Geometry check sheet. Reference: the model listing, model coordinates, mm. Face numbers are marked on the shaded views. A direction names the side the tool comes from. Coordinates: 2 decimals unless noted, no trailing zeros. Loops run counter-clockwise (first coordinate to the right, second up) from the corner with the lowest first, then second, coordinate; pieces in that order, holes last. Notation, with made-up numbers: M 5,66.25 L 38,66.25 A16 cw 38,87.25 Z; hole C 34.25,81.25 d5. An arc over 180 degrees is marked long. Use CSV: the item, a comma, the result in double quotes.
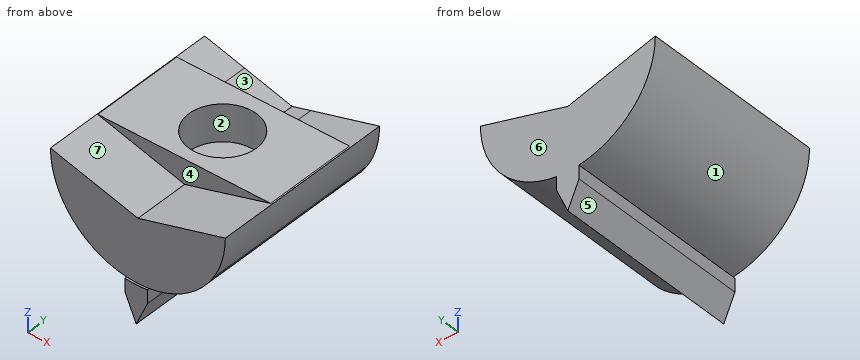
```python
from build123d import *

# Parameters (mm, degrees)
F1_DEPTH = 127
F3_DEPTH = 128.4378021955
F5_DEPTH = 88.5605067015
F6_DEPTH = 23.5462002456
F7_R     = 23.3912457605
F8_DEPTH = 25.4


with BuildPart() as f1:
    # F0 (on Front) → F1 (new body)
    with BuildSketch(Plane.XZ):
        with BuildLine():
            Line((0.0581891033, -16.9071952176), (-60.6434829533, 0))
            ThreePointArc((-60.6434829533, 0), (-58.419745585, -16.2716117976), (-51.9116180406, -31.3498953286))
            Line((-51.9116180406, -31.3498953286), (0.0581891033, -16.9071952176))
        make_face()
        with BuildLine():
            Line((51.9116180406, -31.3498953286), (-51.9116180406, -31.3498953286))
            ThreePointArc((-51.9116180406, -31.3498953286), (0, -60.6434829533), (51.9116180406, -31.3498953286))
        make_face()
        Polygon((0.0581891033, -16.9071952176), (-51.9116180406, -31.3498953286), (51.9116180406, -31.3498953286), align=None)
        with BuildLine():
            Line((60.6434423053, -0.0702144545), (0.0581891033, -16.9071952176))
            Line((0.0581891033, -16.9071952176), (51.9116180406, -31.3498953286))
            ThreePointArc((51.9116180406, -31.3498953286), (58.4103159662, -16.3054289561), (60.6434423053, -0.0702144545))
        make_face()
    extrude(amount=F1_DEPTH)

    # F2 (on face) → F3 (join)
    with BuildSketch(Plane(origin=(0, 0, 0), x_dir=(-1, 0, 0), z_dir=(0, 1, 0))):
        with BuildLine():
            Line((-7.8074381221, -60.1388055641), (-7.8074381221, -69.4347918034))
            Line((-7.8074381221, -69.4347918034), (7.6910599156, -69.4347918034))
            Line((7.6910599156, -69.4347918034), (7.6910599156, -60.1537997311))
            ThreePointArc((7.6910599156, -60.153799731), (-0.0586700775, -60.6434545729), (-7.8074381221, -60.1388055641))
        make_face()
        Polygon((7.6910599156, -69.4347918034), (-7.8074381221, -69.4347918034), (-0.0581891033, -86.9502127171), align=None)
    extrude(amount=-F3_DEPTH)

    # F4 (on Front) → F5 (join)
    with BuildSketch(Plane.XZ):
        Polygon((59.6265792847, 0), (0, 0), (0, -17.0218236744), align=None)
        Polygon((0, -17.0218236744), (0, 0), (-60.2563172579, 0), align=None)
    extrude(amount=F5_DEPTH)

    # F4 (on Front) → F6 (cut)
    with BuildSketch(Plane.XZ):
        Polygon((59.6265792847, 0), (0, 0), (0, -17.0218236744), align=None)
        Polygon((0, -17.0218236744), (0, 0), (-60.2563172579, 0), align=None)
    extrude(amount=F6_DEPTH, mode=Mode.SUBTRACT)

    # F7 (on face) → F8 (cut)
    with BuildSketch(Plane.XY):
        with Locations((-0.3148689866, -56.783683598)):
            Circle(F7_R)
    extrude(amount=-F8_DEPTH, mode=Mode.SUBTRACT)


solid = f1.part
```
1. Section check B-B, the plane y = -98. Record the cut outline in (x, z), plus the area to 3 significant figures.
The answers:
outline,"M -60.64,0 A60.64 ccw -7.69,-60.15 L -7.69,-69.43 L 0.06,-86.95 L 7.81,-69.43 L 7.81,-60.14 A60.64 ccw 60.64,-0.07 L 0.06,-16.91 Z"
area,"5,020 mm^2"
2. Section check A-A, the plane x = -43.5. Record the cut outline in (y, z), plus the area to 3 significant figures.
The answers:
outline,"M -127,-42.25 L 0,-42.25 L 0,-4.77 L -127,-4.77 Z; M -88.56,-4.73 L -23.55,-4.73 L -23.55,0 L -88.56,0 Z"
area,"5,070 mm^2"
3. Gauge pin test, flat ends, axial feed: P1, Ø8.5, axis at x = -24, z = -5.5, coming from the +Y side; P2, Ø6, axis at y = -111.5, z = -23, coming from the +X side; P3, Ø4, axis at y = -23.5, z = -71.5, coming from the -X side. Record the tip position at first contact, or that the pin passes through.
The answers:
P1,"y = -23.55"
P2,"x = 57.25"
P3,"x = -7.66"
4. Set-up check for the marked faces 1, 2, 3 and 4: record each of +Z, -Z, +X, -X, +Y, -Y from which the full face is reachable in a straight line by a thin tool's end or side.
The answers:
face 1,"-Z, -X, +Y, -Y"
face 2,"+Z"
face 3,"+Z, +Y"
face 4,"+Z, -Y"
5. Thickness scan on line 1 (Y direction, x = 35.5, z = -21); line 2 (Z direction, x = 45, y = -85.5); line 3 (Y direction, x = -28, z = -4.5). Record the ranges inside material, lowest first. Write a range as [from, to].
The answers:
line 1,"[-127, 0]"
line 2,"[-40.65, -4.42], [-4.18, 0]"
line 3,"[-88.56, -23.55]"
6. Section check C-C, the plane x = -21. Record the cut outline in (y, z), plus the area to 3 significant figures.
The answers:
outline,"M -127,-56.89 L 0,-56.89 L 0,-11.09 L -23.55,-11.09 L -23.55,0 L -45.86,0 L -45.86,-25.4 L -67.71,-25.4 L -67.71,0 L -88.56,0 L -88.56,-11.04 L -127,-11.04 Z"
area,"5,980 mm^2"
7. Section check D-D, the plane z = -55. Record the cut outline in (x, y), plus the area to 3 significant figures.
The answers:
outline,"M -25.55,-127 L 25.55,-127 L 25.55,0 L -25.55,0 Z"
area,"6,490 mm^2"
8. Release check for a two-part mould opening along X. For the marked faces 5, 6 and 7 record: +X half, -X half, draft (parallel to the pull), parting line (faces both ways), or undercut.
The answers:
face 5,"-X half"
face 6,"draft"
face 7,"undercut"
